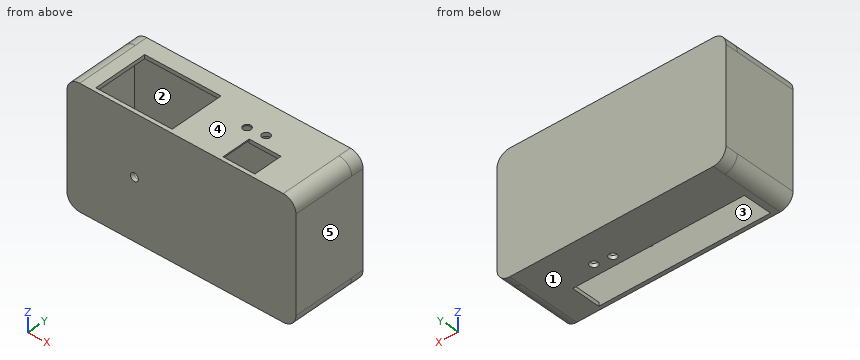
from build123d import *

# Parameters (mm, degrees)
SKETCH1_W           = 45.72
SKETCH1_H           = 24.13
BOSS_EXTRUDE1_DEPTH = 12.446
SHELL2_T            = -0.762
SKETCH2_W           = 22.606
SKETCH2_H           = 10.922
BOSS_EXTRUDE2_DEPTH = 0.762
FILLET1_R           = 2.54
SKETCH4_W           = 34.29
SKETCH4_H           = 3.81
SKETCH4_W_2         = 15.24
SKETCH4_H_2         = 2.54
CUT_EXTRUDE2_DEPTH  = 10.922
SKETCH6_W           = 6.35
SKETCH6_H           = 1.27
CUT_EXTRUDE3_DEPTH  = 10.922
SKETCH7_W           = 10.16
SKETCH7_H           = 10.922
CUT_EXTRUDE4_DEPTH  = 0.508
SKETCH8_R           = 3.175
SKETCH8_R_2         = 0.79375
BOSS_EXTRUDE3_DEPTH = 3.81
SKETCH9_R           = 1.27
SKETCH9_R_2         = 0.381
BOSS_EXTRUDE4_DEPTH = 2.286
CUT_EXTRUDE5_REACH  = 55.174
SKETCH10_R          = 0.79375
SKETCH10_R_2        = 0.381
BOSS_EXTRUDE5_START = -0.762
SKETCH11_R          = 0.381
BOSS_EXTRUDE5_DEPTH = 0.762
SKETCH12_R          = 0.79375
CUT_EXTRUDE6_DEPTH  = 0.762
SKETCH13_W          = 34.29
SKETCH13_H          = 5.08
BOSS_EXTRUDE6_DEPTH = 0.762
SKETCH14_R          = 0.79375
CUT_EXTRUDE7_DEPTH  = 54.174037048
BOSS_EXTRUDE7_START = 2.54
BOSS_EXTRUDE7_DEPTH = 2.54
SKETCH16_W          = 44.196
SKETCH16_H          = 22.606
CUT_EXTRUDE9_DEPTH  = 2.54
SKETCH18_W          = 6.35
SKETCH18_H          = 5.08
SKETCH18_R          = 0.79375
BOSS_EXTRUDE8_DEPTH = 0.762
CUT_EXTRUDE12_START = -2.54
SKETCH19_R          = 0.79375
CUT_EXTRUDE12_DEPTH = 2.54


with BuildPart() as part:
    # Sketch1 → Boss-Extrude1 (new body)
    with BuildSketch(Plane(origin=(0, 0, 0), x_dir=(1, 0, 0), z_dir=(0, 1, 0))):
        with Locations((22.86, 12.065)):
            Rectangle(SKETCH1_W, SKETCH1_H)
    extrude(amount=BOSS_EXTRUDE1_DEPTH)

    # Shell2
    shell2_openings = [part.faces().sort_by_distance(p)[0] for p in [
        (0, 6.223, -12.065),
    ]]
    offset(amount=SHELL2_T, openings=shell2_openings, kind=Kind.INTERSECTION)

    # Sketch2 → Boss-Extrude2 (add)
    with BuildSketch(Plane.ZY):
        with Locations((-12.065, 6.223)):
            Rectangle(SKETCH2_W, SKETCH2_H)
    extrude(amount=-BOSS_EXTRUDE2_DEPTH)

    # Fillet1
    fillet1_edges = [part.edges().sort_by_distance(p)[0] for p in [
        (0, 6.223, -24.13),
        (45.72, 6.223, -24.13),
        (45.72, 6.223, 0),
        (0, 6.223, 0),
    ]]
    fillet(fillet1_edges, radius=FILLET1_R)

    # Sketch4 → Cut-Extrude2 (cut)
    with BuildSketch(Plane(origin=(0, 0.762, 0), x_dir=(1, 0, 0), z_dir=(0, 1, 0))):
        with Locations((20.955, 23.495)):
            Rectangle(SKETCH4_W, SKETCH4_H)
        with Locations((12.7, 0)):
            Rectangle(SKETCH4_W_2, SKETCH4_H_2)
    extrude(amount=CUT_EXTRUDE2_DEPTH, mode=Mode.SUBTRACT)

    # Sketch6 → Cut-Extrude3 (cut)
    with BuildSketch(Plane(origin=(0, 0.762, 0), x_dir=(1, 0, 0), z_dir=(0, 1, 0))):
        with Locations((33.655, 0.635)):
            Rectangle(SKETCH6_W, SKETCH6_H)
    extrude(amount=CUT_EXTRUDE3_DEPTH, mode=Mode.SUBTRACT)

    # Sketch7 → Cut-Extrude4 (cut)
    with BuildSketch(Plane(origin=(0, 0, -0.762), x_dir=(-1, 0, 0), z_dir=(0, 0, -1))):
        with Locations((-25.4, 6.223)):
            Rectangle(SKETCH7_W, SKETCH7_H)
    extrude(amount=-CUT_EXTRUDE4_DEPTH, mode=Mode.SUBTRACT)

    # Sketch8 → Boss-Extrude3 (add)
    with BuildSketch(Plane(origin=(0, 0.762, 0), x_dir=(1, 0, 0), z_dir=(0, 1, 0))):
        with Locations(Location((13.462, 12.065, 0), (0, 0, 90))):
            Circle(SKETCH8_R)
        with Locations(Location((13.462, 12.065, 0), (0, 0, 90))):
            Circle(SKETCH8_R_2, mode=Mode.SUBTRACT)
    extrude(amount=BOSS_EXTRUDE3_DEPTH)

    # Sketch9 → Boss-Extrude4 (add)
    with BuildSketch(Plane(origin=(0, 0.762, 0), x_dir=(1, 0, 0), z_dir=(0, 1, 0))):
        with Locations(Location((27.50252945, 16.967141741, 0), (0, 0, 90))):
            Circle(SKETCH9_R)
        with Locations(Location((27.50252945, 16.967141741, 0), (0, 0, 270))):
            Circle(SKETCH9_R_2, mode=Mode.SUBTRACT)
    extrude(amount=BOSS_EXTRUDE4_DEPTH)

    # Sketch10 → Cut-Extrude5 (cut, up to next)
    with BuildSketch(Plane.XZ, mode=Mode.PRIVATE) as cut_extrude5_sk1:
        with Locations(Location((13.462, -12.065, 0), (0, 0, 270))):
            Circle(SKETCH10_R)
    cut_extrude5_tool1 = extrude(cut_extrude5_sk1.sketch, amount=-CUT_EXTRUDE5_REACH, mode=Mode.PRIVATE) & part.part
    # Sketch10 → Cut-Extrude5 (cut, up to next)
    with BuildSketch(Plane.XZ, mode=Mode.PRIVATE) as cut_extrude5_sk2:
        with Locations(Location((27.50252945, -16.967141741, 0), (0, 0, 270))):
            Circle(SKETCH10_R_2)
    cut_extrude5_tool2 = extrude(cut_extrude5_sk2.sketch, amount=-CUT_EXTRUDE5_REACH, mode=Mode.PRIVATE) & part.part
    # Sketch10 → Cut-Extrude5 (cut, up to next)
    with BuildSketch(Plane.XZ, mode=Mode.PRIVATE) as cut_extrude5_sk3:
        with Locations(Location((33.344788808, -6.833988408, 0), (0, 0, 270))):
            Circle(SKETCH10_R_2)
    cut_extrude5_tool3 = extrude(cut_extrude5_sk3.sketch, amount=-CUT_EXTRUDE5_REACH, mode=Mode.PRIVATE) & part.part
    add(cut_extrude5_tool1.solids().sort_by_distance((13.462, 0, -12.065))[0], mode=Mode.SUBTRACT)
    add(cut_extrude5_tool2.solids().sort_by_distance((27.502529, 0, -16.967142))[0], mode=Mode.SUBTRACT)
    add(cut_extrude5_tool3.solids().sort_by_distance((33.344789, 0, -6.833988))[0], mode=Mode.SUBTRACT)

    # Sketch11 → Boss-Extrude5 (add)
    with BuildSketch(Plane.XZ.offset(BOSS_EXTRUDE5_START)):
        with Locations(Location((27.50252945, -16.967141741, 0), (0, 0, 270))):
            Circle(SKETCH11_R)
        with Locations((33.344788808, -6.833988408)):
            Circle(SKETCH11_R)
    extrude(amount=BOSS_EXTRUDE5_DEPTH)

    # Sketch12 → Cut-Extrude6 (cut)
    with BuildSketch(Plane.XY):
        with Locations((28.36322115, 8.4984082)):
            Circle(SKETCH12_R)
    extrude(amount=-CUT_EXTRUDE6_DEPTH, mode=Mode.SUBTRACT)

    # Sketch13 → Boss-Extrude6 (add)
    with BuildSketch(Plane(origin=(0, 0, -24.13), x_dir=(-1, 0, 0), z_dir=(0, 0, -1))):
        with Locations((-20.955, 9.144)):
            Rectangle(SKETCH13_W, SKETCH13_H)
    extrude(amount=-BOSS_EXTRUDE6_DEPTH)

    # Sketch14 → Cut-Extrude7 (cut, through all)
    with BuildSketch(Plane(origin=(0, 0, -24.13), x_dir=(-1, 0, 0), z_dir=(0, 0, -1))):
        with Locations(Location((-28.36322115, 8.4984082, 0), (0, 0, 180))):
            Circle(SKETCH14_R)
    extrude(amount=-CUT_EXTRUDE7_DEPTH, mode=Mode.SUBTRACT)

    # Sketch15 → Boss-Extrude7 (add)
    with BuildSketch(Plane(origin=(0, 12.446, 0), x_dir=(1, 0, 0), z_dir=(0, 1, 0)).offset(BOSS_EXTRUDE7_START)):
        with BuildLine():
            Line((0, 2.54), (0, 21.59))
            ThreePointArc((0, 21.59), (0.743948776, 23.386051224), (2.54, 24.13))
            Line((2.54, 24.13), (43.18, 24.13))
            ThreePointArc((43.18, 24.13), (44.976051224, 23.386051224), (45.72, 21.59))
            Line((45.72, 21.59), (45.72, 2.54))
            ThreePointArc((45.72, 2.54), (44.976051224, 0.743948776), (43.18, 0))
            Line((43.18, 0), (2.54, 0))
            ThreePointArc((2.54, 0), (0.743948776, 0.743948776), (0, 2.54))
        make_face()
    extrude(amount=-BOSS_EXTRUDE7_DEPTH)

    # Sketch16 → Cut-Extrude9 (cut)
    with BuildSketch(Plane.XZ.offset(-11.684)):
        with Locations((22.86, -12.065)):
            Rectangle(SKETCH16_W, SKETCH16_H)
    extrude(amount=-CUT_EXTRUDE9_DEPTH, mode=Mode.SUBTRACT)

    # Sketch18 → Boss-Extrude8 (add)
    with BuildSketch(Plane.XY):
        with Locations((33.655, 9.144)):
            Rectangle(SKETCH18_W, SKETCH18_H)
        with Locations((31.786109402, 8.930211756)):
            Circle(SKETCH18_R, mode=Mode.SUBTRACT)
    extrude(amount=-BOSS_EXTRUDE8_DEPTH)

    # Sketch19 → Cut-Extrude12 (cut)
    with BuildSketch(Plane(origin=(0, 0, -24.13), x_dir=(-1, 0, 0), z_dir=(0, 0, -1)).offset(CUT_EXTRUDE12_START)):
        with Locations(Location((-31.786109402, 8.930211756, 0), (0, 0, 180))):
            Circle(SKETCH19_R)
    extrude(amount=CUT_EXTRUDE12_DEPTH, mode=Mode.SUBTRACT)


solid = part.part
CAD build for the part. Positions are in the model's coordinates, mm. Face numbers are marked on the shaded views. A direction names the side the tool comes from. Give positions to 0.01 mm unless a question says otherwise; leave off trailing zeros. Write each loop counter-clockwise with the first axis right and the second up, starting at its lowest first coordinate (ties: lowest second). Pieces come first, ordered by that corner, then holes. Notation, with made-up numbers: (76.5, 72) - (123.5, 72) arc R18 cw to (123.5, 86) - close; hole circle Ø8 at (38, 37.25). An arc over 180 degrees is marked (long way). Put each result on its own line as item: value.
(1) Pull direction X, two halves, no side cores. Call the marked faces 3, 4 and 5: released by +X, released by -X, zero draft, split by the parting line, or undercut.
Working result:
face 3: undercut
face 4: zero draft
face 5: released by +X
(2) Drop flat-ended pins along their axis: pin 1 Ø2 at (x, y) = (36, 4.5) entering from -Z; pin 2 Ø6.5 at (x, y) = (13, 5.5) entering from +Z; pin 3 Ø0.6 at (y, z) = (4, -24) entering from -X. Give the stop position or say it passes through.
Working result:
pin 1: z = -0.76
pin 2: z = -8.89
pin 3: x = 1.13
(3) Saw through at A-A (x = 34). List the corners of the cut face in (y, z).
Working result:
outline: (0, -24.13) - (0.76, -24.13) - (0.76, 0) - (0, 0) - close; (6.6, -24.13) - (14.99, -24.13) - (14.99, 0) - (6.6, 0) - (6.6, -0.76) - (14.22, -0.76) - (14.22, -23.37) - (6.6, -23.37) - close
(4) Saw through at B-B (z = -21). List the corners of the cut face in (x, y).
Working result:
outline: (0, 0) - (45.72, 0) - (45.72, 14.99) - (0, 14.99) - close; hole (0.76, 0.76) - (44.96, 0.76) - (44.96, 14.22) - (0.76, 14.22) - close
(5) Saw through at D-D (x = 8.5). List the corners of the cut face in (y, z), then the cut area to 3 significant figures.
Working result:
outline: (0, -24.13) - (0.76, -24.13) - (0.76, 0) - (0, 0) - close; (6.6, -24.13) - (14.99, -24.13) - (14.99, 0) - (11.68, 0) - (11.68, -0.76) - (14.22, -0.76) - (14.22, -23.37) - (6.6, -23.37) - close
area: 44.5 mm^2
(6) Wall check: L1, parallel to Y at x = 8, z = -12; L2, parallel to X at y = 8.5, z = -15.25; L3, parallel to Z at x = 25.5, y = 12.25. Give the ranges that are in metal, low to high.
Working result:
L1: 0 to 0.76, 14.22 to 14.99
L2: 0 to 0.76, 44.96 to 45.72
L3: -24.13 to -23.37, -0.76 to 0
(7) Tool access for the marked faces 1 and 2: list every direction of +Z, -Z, +X, -X, +Y, -Y with a clear straight run to the whole face (end or side of a thin tool).
Working result:
face 1: -Z, +X, -X, +Y, -Y
face 2: none
(8) Saw through at C-C (x = 3). List the corners of the cut face in (y, z), then the cut area to 3 significant figures.
Working result:
outline: (0, -24.13) - (14.99, -24.13) - (14.99, 0) - (0, 0) - close; hole (0.76, -23.37) - (14.22, -23.37) - (14.22, -0.76) - (0.76, -0.76) - close
area: 57.3 mm^2
